```python
from build123d import *

# Parameters (mm, degrees)
CHAMFER1_SIZE      = 0.22
CHAMFER1_SIZE2     = 0.381051178
CUT_EXTRUDE1_DEPTH = 0.85
CUT_EXTRUDE1_TAPER = 6


with BuildPart() as part:
    # Sketch1 → Revolve1 (revolve)
    with BuildSketch(Plane.XY):
        with BuildLine():
            Line((0, 2), (-0.897999199, 2))
            ThreePointArc((-0.897999199, 2), (-1.419403703, 1.059811908), (-1.6, 0))
            Line((-1.6, 0), (6.5, 0))
            Line((6.5, 0), (6.5, 1.1))
            Line((6.5, 1.1), (0, 1.1))
            Line((0, 1.1), (0, 2))
        make_face()
    revolve(axis=Axis((0, 0, 0), (1, 0, 0)))

    # Chamfer1
    chamfer1_edges = [part.edges().sort_by_distance(p)[0] for p in [
        (6.5, -1.1, 0),
    ]]
    chamfer1_side = [part.faces().sort_by_distance(p)[0] for p in [
        (6.5, 0, 0),
    ]]
    chamfer(chamfer1_edges, length=CHAMFER1_SIZE, length2=CHAMFER1_SIZE2, reference=chamfer1_side[0])

    # Sketch2 → EndCone (revolve, cut)
    with BuildSketch(Plane.XY):
        Polygon((6.5, 0), (4.594744112, 1.1), (4.594744112, 1.2), (6.6, 1.2), (6.6, 0), align=None)
    revolve(axis=Axis((0, 0, 0), (1, 0, 0)), mode=Mode.SUBTRACT)

    # Sketch3 → Cut-Extrude1 (cut)
    with BuildSketch(Plane(origin=(-1.6, 0, 0), x_dir=(0, 0, -1), z_dir=(1, 0, 0))):
        Polygon((-0.2375, 0.95), (-0.1425, 0.57), (-0.29897586, 0.29897586), (-0.57, 0.1425), (-0.95, 0.2375), (-0.95, -0.2375), (-0.57, -0.1425), (-0.29897586, -0.29897586), (-0.1425, -0.57), (-0.2375, -0.95), (0.2375, -0.95), (0.1425, -0.57), (0.29897586, -0.29897586), (0.57, -0.1425), (0.95, -0.2375), (0.95, 0.2375), (0.57, 0.1425), (0.29897586, 0.29897586), (0.1425, 0.57), (0.2375, 0.95), align=None)
    extrude(amount=CUT_EXTRUDE1_DEPTH, taper=CUT_EXTRUDE1_TAPER, mode=Mode.SUBTRACT)


solid = part.part
```
Design review of the part built by this model. Coordinates are the model's own, in mm. Coordinates: 2 decimals unless noted, no trailing zeros. Order: outer loops, then holes, each group sorted by start corner. A loop starts at its lowest first (then second) coordinate and runs counter-clockwise, first axis right, second up. Notation, with made-up numbers: (-1, 87) -> (37, 87) arc R8 cw to (37, 92) -> close; hole circle Ø8 at (61.5, 29.5). An arc over 180 degrees is marked (long way). One line per item, written item: value. Start each with the question number.
Q1. Insertion check: pin 1 Ø2 at (x, z) = (2.5, 1) entering from -Y; pin 2 Ø1 at (x, z) = (5.5, 1.5) entering from +Y; pin 3 Ø1.5 at (x, y) = (0.5, 1) entering from -Z. Each pin has a flat end and moves straight along its axis. Give the tip position at first contact, or say it passes through.
Q2. Take a section at B-B, the plane x = 2.75. State the section outline as (y, z) points.
Q3. Take a section at A-A, the plane y = -1.2. State the section outline as (x, z) points, then the cut area to 3 significant figures.
Q4. Mouldability with a two-part tool opening along Z and no side actions: class faces 1 (the cylindrical face through (2.27, 1.05, 0.33)), 2 (the flat face through (0, -1, -1)), 3 (the flat face through (-0.75, 0, 0)) as pulls with the +Z half, pulls with the -Z half, needs draft (parallel to the pull), parting line crosses it, or undercut.
Q5. Take a section at D-D, the plane x = 5.5. State the section outline as (y, z) points.
Q6. Take a section at C-C, the plane z = 1.7. State the section outline as (x, y) points.
Q7. For probe 1 along Y at (x, z) = (-1, -0.3); probe 2 along Z at (x, y) = (4.5, 0.25); probe 3 along Z at (x, y) = (5.25, -0.05), list the stretches that pass through material, from the lowest coordinate up.
Values follow:
1. pin 1: stops at y = -1.1
1. pin 2: passes through
1. pin 3: stops at z = -1.95
2. outline: circle Ø2.2 at (0, 0)
3. outline: (-0.9, -1.6) -> (0, -1.6) -> (0, 1.6) -> (-0.9, 1.6) arc R2.97 ccw to start
3. area: 3.89 mm2
4. face 1: parting line crosses it
4. face 2: needs draft
4. face 3: undercut
5. outline: circle Ø1.15 at (0, 0)
6. outline: (-0.9, -1.05) -> (0, -1.05) -> (0, 1.05) -> (-0.9, 1.05) arc R2.71 ccw to start
7. probe 1: y = -1.84 to -0.23, 0.23 to 1.84
7. probe 2: z = -1.07 to 1.07
7. probe 3: z = -0.72 to 0.72
